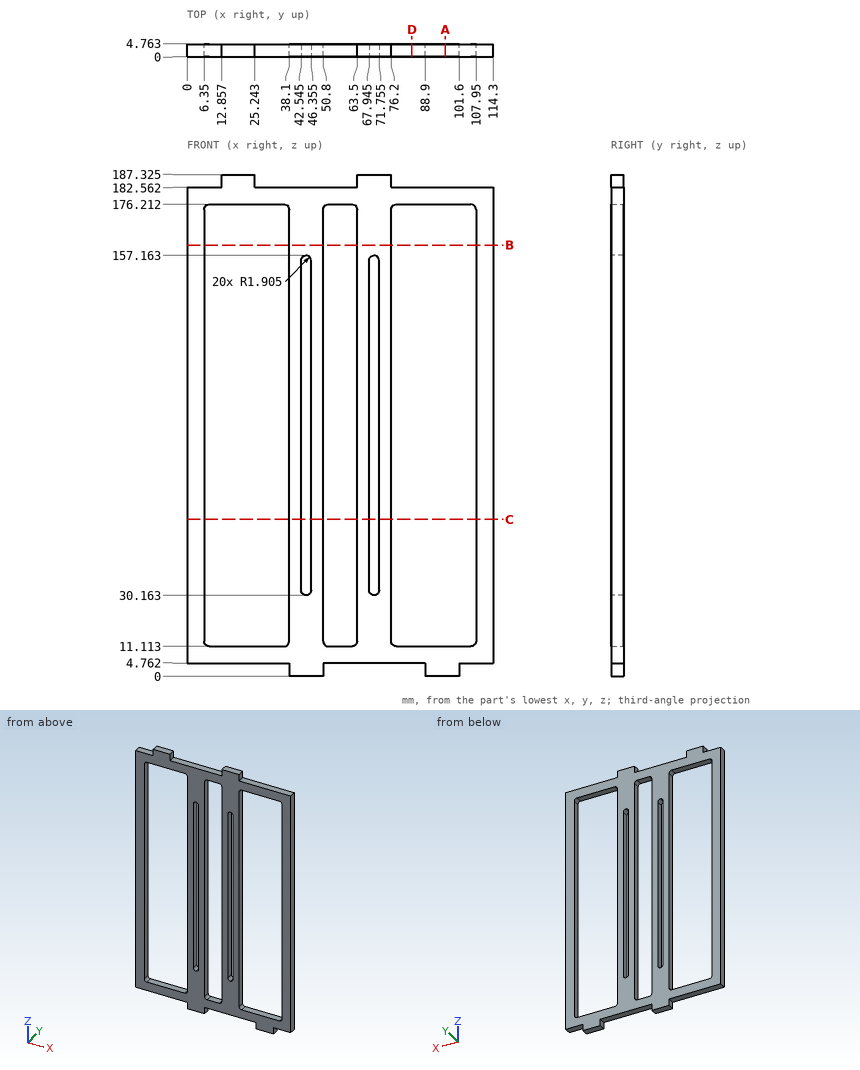
Study the drawing (mm; zero at the part's minimum x, y, z) and answer. Coordinates: 2 decimals unless noted, no trailing zeros. Order: outer loops, then holes, each group sorted by start corner. A loop starts at its lowest first (then second) coordinate and runs counter-clockwise, first axis right, second up. Notation, with made-up numbers: (5.5, 51.25) -> (10.5, 51.25) arc R20 ccw to (10.5, 66.25) -> close; hole circle Ø6 at (-3.75, 19). An arc over 180 degrees is marked (long way). Answer in a Markdown table with one row per item. Add a question column.
Item 1: Find section C-C (z = 58.5). State how many separate pieces and enclosed holes the cut face has, then the cut area to 3 significant figures.
Item 2: Find section A-A (x = 96.5). Write down the section's boundary in (y, z).
Item 3: Each of these flat-tipped pins is pushed along its axis until it touches: P1, Ø1.4, axis at y = 1.5, z = 2, coming from the +X side; P2, Ø2.5, axis at x = 109, y = 3, coming from the -Z side; P3, Ø1, axis at x = 52.5, y = 3.5, coming from the +Z side. Where does it stop, or does it pass through?
Item 4: Find section B-B (z = 161). Write down the section's boundary in (x, y).
Item 5: Find section D-D (x = 84). Write down the section's boundary in (y, z).
Item 6: Find the intervals of material crossed by L1, parallel to X at y = 2, z = 159; L2, parallel to Z at x = 36, y = 3.8; L3, parallel to Z at x = 95, y = 2.4, in increasing order. Write a range as from..to.
Result set:
| question | item | result |
|---|---|---|
| 1 | separate pieces | 6 |
| 1 | enclosed holes | 0 |
| 1 | area | 145 mm² |
| 2 | outline | (0, 0) -> (4.76, 0) -> (4.76, 11.11) -> (0, 11.11) -> close; (0, 176.21) -> (4.76, 176.21) -> (4.76, 182.56) -> (0, 182.56) -> close |
| 3 | P1 | stops at x = 101.6 |
| 3 | P2 | stops at z = 4.76 |
| 3 | P3 | stops at z = 182.56 |
| 4 | outline | (0, 0) -> (6.35, 0) -> (6.35, 4.76) -> (0, 4.76) -> close; (38.1, 0) -> (50.8, 0) -> (50.8, 4.76) -> (38.1, 4.76) -> close; (63.5, 0) -> (76.2, 0) -> (76.2, 4.76) -> (63.5, 4.76) -> close; (107.95, 0) -> (114.3, 0) -> (114.3, 4.76) -> (107.95, 4.76) -> close |
| 5 | outline | (0, 4.76) -> (4.76, 4.76) -> (4.76, 11.11) -> (0, 11.11) -> close; (0, 176.21) -> (4.76, 176.21) -> (4.76, 182.56) -> (0, 182.56) -> close |
| 6 | L1 | x = 0..6.35, 38.1..50.8, 63.5..76.2, 107.95..114.3 |
| 6 | L2 | z = 4.76..11.11, 176.21..182.56 |
| 6 | L3 | z = 0..11.11, 176.21..182.56 |
